from build123d import *

# Parameters (mm, degrees)
PAD001_DEPTH = 10
SKETCH002_R  = 1.8
POCKET_DEPTH = 3.501
SKETCH_W     = 10
SKETCH_H     = 33
SKETCH_R     = 1.8
PAD_DEPTH    = 1.8


with BuildPart() as body001:
    # Sketch001 → Pad001 (new body)
    with BuildSketch(Plane.YZ.offset(-5)):
        Polygon((0, 1.8), (0, 5.3), (6, 5.3), (6, 12.5), (10.65, 12.5), (10.65, 5.3), (13.85, 5.3), (13.85, 12.5), (18.5, 12.5), (18.5, 5.3), (24.5, 5.3), (24.5, 1.8), align=None)
    extrude(amount=PAD001_DEPTH)

    # Sketch002 (on Face2 of Pad001) → Pocket (cut, through all)
    with BuildSketch(Plane(origin=(0, 0, 5.3), x_dir=(0, -1, 0), z_dir=(0, 0, 1))):
        with Locations((-22.36288, 0)):
            Circle(SKETCH002_R)
        with Locations((-3, 0)):
            Circle(SKETCH002_R)
    extrude(amount=-POCKET_DEPTH, mode=Mode.SUBTRACT)


with BuildPart() as fusion:
    # Sketch → Pad (new body)
    with BuildSketch(Plane.XY):
        with Locations((0, 16.5)):
            Rectangle(SKETCH_W, SKETCH_H)
        with Locations((0, 22)):
            Circle(SKETCH_R, mode=Mode.SUBTRACT)
        with Locations((0, 3)):
            Circle(SKETCH_R, mode=Mode.SUBTRACT)
    extrude(amount=PAD_DEPTH)

    # Fusion: union Body001
    add(body001.part)


solid = fusion.part
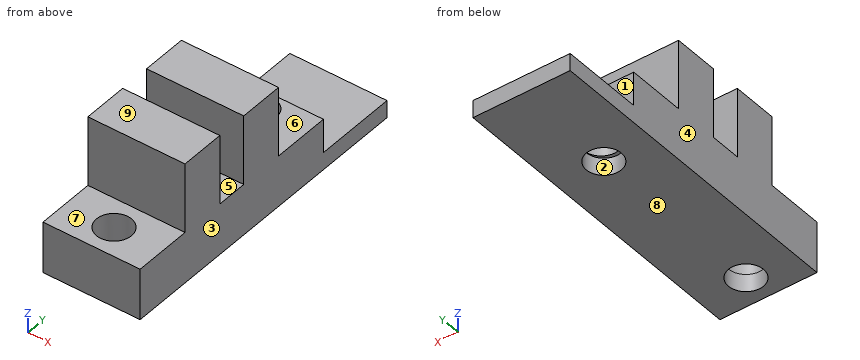
Model file for the job. Use its own axes, mm. Face numbers are marked on the shaded views. A direction names the side the tool comes from. Give positions to 0.01 mm unless a question says otherwise; leave off trailing zeros. Loops run counter-clockwise (first coordinate to the right, second up) from the corner with the lowest first, then second, coordinate; pieces in that order, holes last. Notation, with made-up numbers: (55, 58.5) -> (88, 58.5) arc R27 cw to (88, 76.5) -> close; hole circle Ø5 at (-12, 37). An arc over 180 degrees is marked (long way). Use a Markdown table: item, result. Add a question column.
(1) Drop flat-ended pins along their axis: pin 1 Ø2 at (x, z) = (-0.5, 7) entering from -Y; pin 2 Ø6 at (x, z) = (1.5, 8.5) entering from +Y; pin 3 Ø3 at (x, y) = (2, 20.5) entering from +Z; pin 4 Ø2 at (x, y) = (0, 22.36) entering from -Z. Give the stop position or say it passes through.
(2) Tool access for the marked faces 5, 6, 7, 8 and 9: list every direction of +Z, -Z, +X, -X, +Y, -Y with a clear straight run to the whole face (end or side of a thin tool).
(3) Slice it at D-D on z = 3.5. List the corners of the cut face in (x, y).
(4) Slice it at B-B on z = 9. List the corners of the cut face in (x, y), and give its area (3 significant figures).
(5) Slice it at C-C on y = 3. List the corners of the cut face in (x, z), and give its area (3 significant figures).
(6) Slice it at A-A on x = 0. List the corners of the cut face in (y, z).
(7) Wall check: line 1 along Y through (x, z) = (0, 0.95); line 2 along Y through (x, z) = (-2.75, 6); line 3 along X through (y, z) = (22, 1.15). Give the ranges that are in metal, low to high.
(8) Mould opens along X. For the marked faces 1, 2, 3 and 4 say: +X half, -X half, draft (parallel to the pull), parting line (faces both ways), or undercut.
Filled sheet:
| question | item | result |
|---|---|---|
| 1 | pin 1 | y = 6 |
| 1 | pin 2 | y = 18.5 |
| 1 | pin 3 | z = 5.3 |
| 1 | pin 4 | through |
| 2 | face 5 | +Z, +X, -X |
| 2 | face 6 | +Z, +X, -X, +Y |
| 2 | face 7 | +Z, +X, -X, -Y |
| 2 | face 8 | -Z, +X, -X, +Y, -Y |
| 2 | face 9 | +Z, +X, -X, +Y, -Y |
| 3 | outline | (-5, 0) -> (5, 0) -> (5, 24.5) -> (-5, 24.5) -> close; hole circle Ø3.6 at (0, 3); hole circle Ø3.6 at (0, 22.36) |
| 4 | outline | (-5, 6) -> (5, 6) -> (5, 10.65) -> (-5, 10.65) -> close; (-5, 13.85) -> (5, 13.85) -> (5, 18.5) -> (-5, 18.5) -> close |
| 4 | area | 93.0 mm2 |
| 5 | outline | (-5, 0) -> (-1.8, 0) -> (-1.8, 5.3) -> (-5, 5.3) -> close; (1.8, 0) -> (5, 0) -> (5, 5.3) -> (1.8, 5.3) -> close |
| 5 | area | 33.9 mm2 |
| 6 | outline | (0, 0) -> (1.2, 0) -> (1.2, 5.3) -> (0, 5.3) -> close; (4.8, 0) -> (20.2, 0) -> (20.2, 1.8) -> (20.56, 1.8) -> (20.56, 5.3) -> (18.5, 5.3) -> (18.5, 12.5) -> (13.85, 12.5) -> (13.85, 5.3) -> (10.65, 5.3) -> (10.65, 12.5) -> (6, 12.5) -> (6, 5.3) -> (4.8, 5.3) -> close; (23.8, 0) -> (33, 0) -> (33, 1.8) -> (24.5, 1.8) -> (24.5, 5.3) -> (24.16, 5.3) -> (24.16, 1.8) -> (23.8, 1.8) -> close |
| 7 | line 1 | 0 to 1.2, 4.8 to 20.2, 23.8 to 33 |
| 7 | line 2 | 6 to 10.65, 13.85 to 18.5 |
| 7 | line 3 | -5 to -1.8, 1.8 to 5 |
| 8 | face 1 | draft |
| 8 | face 2 | undercut |
| 8 | face 3 | +X half |
| 8 | face 4 | -X half |
